Geometry check sheet. Reference: drawing and pictorial views, mm from the part's lowest x, y, z. A direction names the side the tool comes from. Coordinates: 2 decimals unless noted, no trailing zeros. Loops run counter-clockwise (first coordinate to the right, second up) from the corner with the lowest first, then second, coordinate; pieces in that order, holes last. Notation, with made-up numbers: (73.5, 36.25) - (89.5, 36.25) arc R16 ccw to (89.5, 44.25) - close; hole circle Ø10 at (-14, 86). An arc over 180 degrees is marked (long way). One line per item, written item: value.
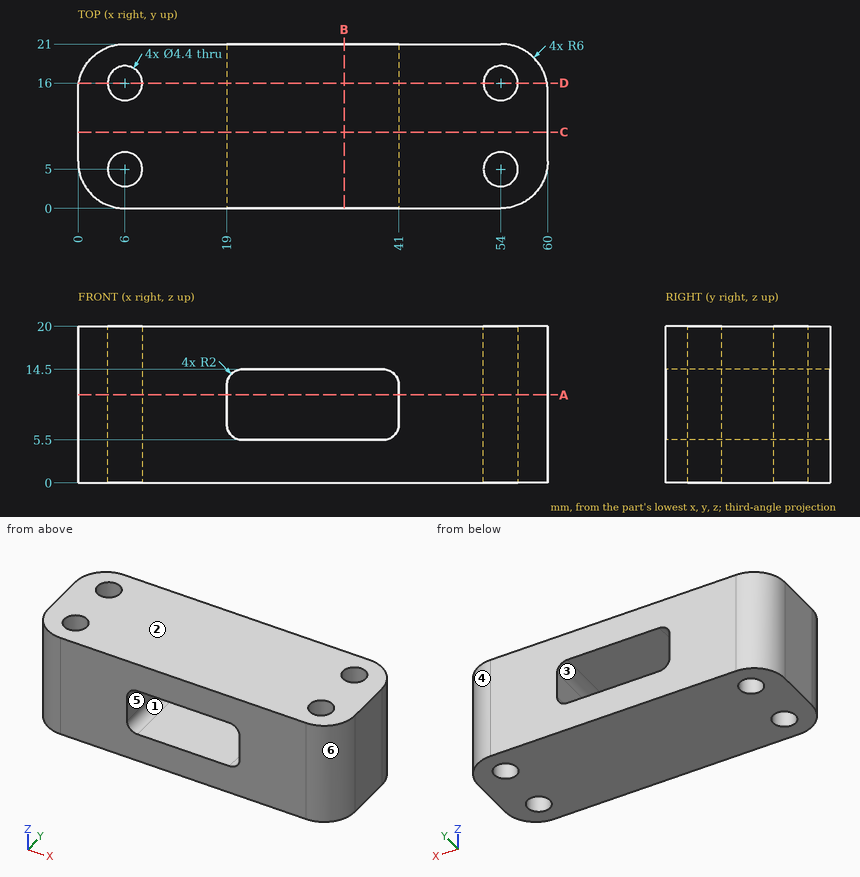
(1) Cross-section at D-D on y = 16. Record the cut outline in (x, z).
Reply:
outline: (0.08, 0) - (3.8, 0) - (3.8, 20) - (0.08, 20) - close; (8.2, 0) - (51.8, 0) - (51.8, 20) - (8.2, 20) - close; (56.2, 0) - (59.92, 0) - (59.92, 20) - (56.2, 20) - close; hole (19, 7.5) arc R2 ccw to (21, 5.5) - (39, 5.5) arc R2 ccw to (41, 7.5) - (41, 12.5) arc R2 ccw to (39, 14.5) - (21, 14.5) arc R2 ccw to (19, 12.5) - close
(2) Material ranges on probe 1 along Y at (x, z) = (6, 13.75); probe 2 along Z at (x, y) = (36.5, 11.5); probe 3 along X at (y, z) = (14.25, 18.75), recorded low to high. Write a range as from..to.
Reply:
probe 1: 0..2.8, 7.2..13.8, 18.2..21
probe 2: 0..5.5, 14.5..20
probe 3: 0..4.67, 7.33..52.67, 55.33..60
(3) Cross-section at A-A on z = 11.25. Record the cut outline in (x, y), and give its area (3 significant figures).
Reply:
outline: (0, 6) arc R6 ccw to (6, 0) - (19, 0) - (19, 21) - (6, 21) arc R6 ccw to (0, 15) - close; (41, 0) - (54, 0) arc R6 ccw to (60, 6) - (60, 15) arc R6 ccw to (54, 21) - (41, 21) - close; hole circle Ø4.4 at (6, 5); hole circle Ø4.4 at (6, 16); hole circle Ø4.4 at (54, 5); hole circle Ø4.4 at (54, 16)
area: 706 mm2
(4) Release check for a two-part mould opening along X. For the marked faces 1, 2, 3 and 4 record: pulls with the +X half, pulls with the -X half, needs draft (parallel to the pull), parting line crosses it, or undercut.
Reply:
face 1: undercut
face 2: needs draft
face 3: undercut
face 4: pulls with the +X half
(5) Cross-section at C-C on y = 9.75. Record the cut outline in (x, z), and give its area (3 significant figures).
Reply:
outline: (0, 0) - (60, 0) - (60, 20) - (0, 20) - close; hole (19, 7.5) arc R2 ccw to (21, 5.5) - (39, 5.5) arc R2 ccw to (41, 7.5) - (41, 12.5) arc R2 ccw to (39, 14.5) - (21, 14.5) arc R2 ccw to (19, 12.5) - close
area: 1,010 mm2
(6) Cross-section at B-B on x = 34. Record the cut outline in (y, z).
Reply:
outline: (0, 0) - (21, 0) - (21, 5.5) - (0, 5.5) - close; (0, 14.5) - (21, 14.5) - (21, 20) - (0, 20) - close
(7) Access from +Z, -Z, +X, -X, +Y, -Y to the whole of each face (thin tool, end or side, straight path). Record for the marked faces 5 and 6.
Reply:
face 5: +Y, -Y
face 6: +Z, -Z, +X, -Y
